```python
from build123d import *

# Parameters (mm, degrees)
SKETCH1_R         = 3.175
EXTRUDE1_DEPTH    = 2.5908
FILLET1_R         = 1.524
SKETCH2_R         = 1.7018
EXTRUDE2_DEPTH    = 8.89
SKETCH3_W         = 3.27637992
SKETCH3_H         = 0.410534548
EXTRUDE3_DEPTH    = 1.016
CIRPATTERN1_COUNT = 2
CIRPATTERN1_ANGLE = 90


with BuildPart() as part:
    # Sketch1 → Extrude1 (new body)
    with BuildSketch(Plane.XY):
        Circle(SKETCH1_R)
    extrude(amount=EXTRUDE1_DEPTH)

    # Fillet1
    fillet1_edges = [part.edges().sort_by_distance(p)[0] for p in [
        (-3.175, 0, 0),
    ]]
    fillet(fillet1_edges, radius=FILLET1_R)

    # Sketch2 → Extrude2 (add)
    with BuildSketch(Plane.XY.offset(2.5908)):
        Circle(SKETCH2_R)
    extrude(amount=EXTRUDE2_DEPTH)

    # Sketch3 → Extrude3 (cut)
    with BuildSketch(Plane(origin=(0, 0, 0), x_dir=(-1, 0, 0), z_dir=(0, 0, -1))):
        Rectangle(SKETCH3_W, SKETCH3_H)
    extrude3 = extrude(amount=-EXTRUDE3_DEPTH, mode=Mode.SUBTRACT)

    # CirPattern1: Extrude3 ×2 about axis
    cirpattern1_axis = Axis((0, 0, 0), (0, 0, -1))
    for i in range(1, CIRPATTERN1_COUNT):
        add(extrude3.rotate(cirpattern1_axis, i * CIRPATTERN1_ANGLE / (CIRPATTERN1_COUNT - 1)), mode=Mode.SUBTRACT)


solid = part.part
```
Check sheet for the modelled part. Datum: model origin and axes. Units: mm. A direction names the side the tool comes from. Coordinates: 2 decimals unless noted, no trailing zeros. Loops run counter-clockwise (first coordinate to the right, second up) from the corner with the lowest first, then second, coordinate; pieces in that order, holes last.
1) Sectioned sample at D-D (z = 2). Record the boundary of the cut face in (x, y) (3 decimals), and give its area (3 significant figures).
2) Release check for a two-part mould opening along X. For faces 1 (the face through (-0.69, -3.1, 2.05)), 2 (the face through (0.9, -0.205, 0.5)), 3 (the face through (1, -1, 0)) record: released by +X, released by -X, zero draft, split by the parting line, or undercut.
3) Access from +Z, -Z, +X, -X, +Y, -Y to the whole of each face (thin tool, end or side, straight path). Record for faces 4 (the face through (-1, 1, 0)), 5 (the face through (1.572, -0.652, 6.974)), 6 (the face through (-0.9, 0.205, 0.5)).
4) Sectioned sample at C-C (z = 9.5). Record the boundary of the cut face in (x, y), and give its area (3 significant figures).
5) Sectioned sample at A-A (x = 0). Record the boundary of the cut face in (y, z) (3 decimals), and give its area (3 significant figures).
6) Material ranges on probe 1 along Z at (x, y) = (0, -1); probe 2 along X at (y, z) = (-0.5, 4.5); probe 3 along Y at (x, z) = (-0.25, 9.5), recorded low to high.
7) Gauge pin test, flat ends, axial feed: pin 1 (0.8 mm diameter, centred on x = 1, z = 0.5, fed in from +Y); pin 2 (0.5 mm diameter, centred on y = 0, z = 0.5, fed in from +X); pin 3 (0.8 mm diameter, centred on y = -1, z = 0.5, fed in from +X); pin 4 (2 mm diameter, centred on x = 1.5, y = 2, fed in from +Z). Record the tip position at first contact, or that the pin passes through.
Check sheet entries:
1. outline: circle Ø6.35 at (0, 0)
1. area: 31.7 mm2
2. face 1: split by the parting line
2. face 2: undercut
2. face 3: zero draft
3. face 4: -Z, +X, -X, +Y, -Y
3. face 5: +Z
3. face 6: -Z
4. outline: circle Ø3.4 at (0, 0)
4. area: 9.10 mm2
5. outline: (-3.175, 1.524) arc R1.524 ccw to (-1.651, 0) - (-1.638, 0) - (-1.638, 1.016) - (1.638, 1.016) - (1.638, 0) - (1.651, 0) arc R1.524 ccw to (3.175, 1.524) - (3.175, 2.591) - (1.702, 2.591) - (1.702, 11.481) - (-1.702, 11.481) - (-1.702, 2.591) - (-3.175, 2.591) - close
5. area: 42.4 mm2
6. probe 1: z = 1.02 to 11.48
6. probe 2: x = -1.63 to 1.63
6. probe 3: y = -1.68 to 1.68
7. pin 1: stops at y = 2.91
7. pin 2: stops at x = 2.96
7. pin 3: stops at x = 2.91
7. pin 4: stops at z = 11.48
